Design review of the part built by this model. Coordinates are the model's own, in mm. A direction names the side the tool comes from. Coordinates: 2 decimals unless noted, no trailing zeros. Loops run counter-clockwise (first coordinate to the right, second up) from the corner with the lowest first, then second, coordinate; pieces in that order, holes last. Notation, with made-up numbers: (-33.75, -1) - (8.25, -1) arc R24 ccw to (8.25, 23) - close; hole circle Ø10 at (76, 82.5). An arc over 180 degrees is marked (long way). Answer in a Markdown table with one row per item. Add a question column.
(1) To check wall thickness, follow L1, parallel to Z at x = -5, y = -4.5; L2, parallel to Z at x = 17, y = -19.5; L3, parallel to X at y = -10.75, z = -19. State the ranges of each line that lie inside material, in increasing order. Write a range as [from, to].
(2) We need section C-C, the plane x = -12. Write out the cut boundary in (y, z).
(3) We need section A-A, the plane x = 0. Write out the cut boundary in (y, z), plus the area to 3 significant figures.
(4) The part is to be moulded in two halves that separate along Z. For faces 1 (the face through (-19, -13, 0)), 2 (the face through (-11.012, -12.522, -49.592)), 3 (the face through (-1, -25.4, 1)), say which applies: released by +Z, released by -Z, zero draft, split by the parting line, or undercut.
(5) For faces 4 (the face through (-1, 0, 1)), 5 (the face through (18, -13, 0)), list the 3-axis set-ups (+Z, -Z, +X, -X, +Y, -Y) from which the entire face can be reached by the end or side of a thin tool; tool diameter is ignored.
(6) We need section B-B, the plane y = -2.5. Write out the cut boundary in (x, z).
(7) We need section D-D, the plane z = 20.5. Write out the cut boundary in (x, y).
(8) Clearance check with flat-ended pins moving along their axes: pin 1 (5 mm diameter, centred on x = -0.5, y = -6.5, fed in from +Z); pin 2 (1.1 mm diameter, centred on y = -11.5, z = 1, fed in from -X); pin 3 (5 mm diameter, centred on y = -14.5, z = -15.5, fed in from +X). State where each tip first meets the part, or that it passes through.
from build123d import *

# Parameters (mm, degrees)
F0_R     = 50.8
F0_W     = 22.86
F0_H     = 2.286
F1_DEPTH = 25.4


with BuildPart() as f1:
    # F0 (on Front) → F1 (new body)
    with BuildSketch(Plane.XZ):
        Circle(F0_R)
        with BuildLine():
            Line((9.832879, -14.010016), (-7.947121, -14.010016))
            ThreePointArc((-7.947121, -14.010016), (0.942879, -8.589429), (9.832879, -14.010016))
        make_face(mode=Mode.SUBTRACT)
        with Locations((-19.05, 1.143)):
            Rectangle(F0_W, F0_H, mode=Mode.SUBTRACT)
        with Locations((18.03015, 1.143)):
            Rectangle(F0_W, F0_H, mode=Mode.SUBTRACT)
    extrude(amount=F1_DEPTH)


solid = f1.part
Responses:
| question | item | result |
|---|---|---|
| 1 | L1 | z = [-50.55, -14.01], [-10.55, 50.55] |
| 1 | L2 | z = [-47.87, 0], [2.29, 47.87] |
| 1 | L3 | x = [-47.11, 47.11] |
| 2 | outline | (-25.4, -49.36) - (0, -49.36) - (0, 0) - (-25.4, 0) - close; (-25.4, 2.29) - (0, 2.29) - (0, 49.36) - (-25.4, 49.36) - close |
| 3 | outline | (-25.4, -50.8) - (0, -50.8) - (0, -14.01) - (-25.4, -14.01) - close; (-25.4, -8.63) - (0, -8.63) - (0, 50.8) - (-25.4, 50.8) - close |
| 3 | area | 2,440 mm2 |
| 4 | face 1 | undercut |
| 4 | face 2 | split by the parting line |
| 4 | face 3 | zero draft |
| 5 | face 4 | +Z, -Z, +X, -X, +Y |
| 5 | face 5 | +Y, -Y |
| 6 | outline | circle Ø101.6 at (0, 0); hole (-30.48, 0) - (-7.62, 0) - (-7.62, 2.29) - (-30.48, 2.29) - close; hole (-7.95, -14.01) - (9.83, -14.01) arc R10 ccw to start; hole (6.6, 0) - (29.46, 0) - (29.46, 2.29) - (6.6, 2.29) - close |
| 7 | outline | (-46.48, -25.4) - (46.48, -25.4) - (46.48, 0) - (-46.48, 0) - close |
| 8 | pin 1 | stops at z = 50.8 |
| 8 | pin 2 | stops at x = -50.8 |
| 8 | pin 3 | stops at x = 49.11 |
